```python
from build123d import *

# Parameters (mm, degrees)
SCHIZZO1_R                    = 2
ESTRUSIONE_ESTRUSIONE1_DEPTH  = 3
ESTRUSIONE_ESTRUSIONE2_DEPTH  = 3
SCHIZZO3_W                    = 5
SCHIZZO3_H                    = 5
ESTRUSIONE_ESTRUSIONE3_DEPTH  = 47
SCHIZZO4_R                    = 1.25
TAGLIO_ESTRUSIONE1_DEPTH      = 15
ESTRUSIONE_ESTRUSIONE4_DEPTH  = 5
ESTRUSIONE_ESTRUSIONE5_DEPTH  = 5
SCHIZZO9_W                    = 50
SCHIZZO9_H                    = 46
ESTRUSIONE_ESTRUSIONE8_DEPTH  = 3
SMUSSO1_SIZE                  = 5
SCHIZZO11_W                   = 17
SCHIZZO11_H                   = 46
SCHIZZO11_W_2                 = 64
SCHIZZO11_H_2                 = 58
TAGLIO_ESTRUSIONE3_DEPTH      = 10
SCHIZZO12_W                   = 60
SCHIZZO12_H                   = 20
TAGLIO_ESTRUSIONE4_DEPTH      = 60
SCHIZZO13_W                   = 27
SCHIZZO13_H                   = 46
TAGLIO_ESTRUSIONE5_DEPTH      = 10
RACCORDO1_R                   = 10
SCHIZZO14_W                   = 8
SCHIZZO14_H                   = 14
ESTRUSIONE_ESTRUSIONE9_DEPTH  = 45
SCHIZZO15_R                   = 1.85
TAGLIO_ESTRUSIONE6_DEPTH      = 20
SCHIZZO16_W                   = 8
SCHIZZO16_H                   = 8
ESTRUSIONE_ESTRUSIONE10_DEPTH = 15
SCHIZZO17_R                   = 1.85
TAGLIO_ESTRUSIONE7_DEPTH      = 15
SCHIZZO18_W                   = 8
SCHIZZO18_H                   = 8
ESTRUSIONE_ESTRUSIONE11_DEPTH = 41
SMUSSO3_SIZE                  = 5
SCHIZZO19_W                   = 8
SCHIZZO19_H                   = 58
ESTRUSIONE_ESTRUSIONE12_DEPTH = 3
RACCORDO2_R                   = 10
SCHIZZO20_R                   = 1.85
TAGLIO_ESTRUSIONE8_DEPTH      = 15
SCHIZZO21_W                   = 80
SCHIZZO21_H                   = 6
TAGLIO_ESTRUSIONE9_DEPTH      = 30
SMUSSO4_SIZE                  = 5
ESTRUSIONE_ESTRUSIONE13_DEPTH = 2
SCHIZZO23_W                   = 5
SCHIZZO23_H                   = 2
TAGLIO_ESTRUSIONE10_DEPTH     = 15
SMUSSO5_SIZE                  = 2
ESTRUSIONE_ESTRUSIONE14_DEPTH = 2


with BuildPart() as part:
    # Schizzo1 → Estrusione-Estrusione1 (new body)
    with BuildSketch(Plane.XY):
        with BuildLine():
            Line((4, 70), (4, 27))
            Line((4, 27), (52, 27))
            Line((52, 27), (52, 18))
            Line((52, 18), (4, 18))
            Line((4, 18), (4, -16))
            Line((4, -16), (52, -16))
            Line((52, -16), (52, -24))
            Line((52, -24), (4, -24))
            Line((4, -24), (4, -67))
            ThreePointArc((4, -67), (0, -71), (-4, -67))
            Line((-4, -67), (-4, -24))
            Line((-4, -24), (-52, -24))
            Line((-52, -24), (-52, -16))
            Line((-52, -16), (-4, -16))
            Line((-4, -16), (-4, 18))
            Line((-4, 18), (-52, 18))
            Line((-52, 18), (-52, 27))
            Line((-52, 27), (-4, 27))
            Line((-4, 27), (-4, 70))
            ThreePointArc((-4, 70), (0, 74), (4, 70))
        make_face()
        with Locations((0, 70)):
            Circle(SCHIZZO1_R, mode=Mode.SUBTRACT)
        with Locations((48, 23)):
            Circle(SCHIZZO1_R, mode=Mode.SUBTRACT)
        with Locations((-48, 23)):
            Circle(SCHIZZO1_R, mode=Mode.SUBTRACT)
        with Locations((0, -67)):
            Circle(SCHIZZO1_R, mode=Mode.SUBTRACT)
        with Locations((-48, -20)):
            Circle(SCHIZZO1_R, mode=Mode.SUBTRACT)
        with Locations((48, -20)):
            Circle(SCHIZZO1_R, mode=Mode.SUBTRACT)
    extrude(amount=ESTRUSIONE_ESTRUSIONE1_DEPTH)

    # Schizzo2 → Estrusione-Estrusione2 (add)
    with BuildSketch(Plane.XY):
        Polygon((-42, 57), (-3.921210291, 57), (-3.921210291, 64), (-49, 64), (-49, 26), (-42, 26), align=None)
        Polygon((-49, 4), (-40, 4), (-40, -62), (40, -62), (40, 4), (49, 4), (49, 18), (42, 18), (42, 11), (3.990161704, 11), (3.990161704, 4), (32, 4), (32, -54), (-32, -54), (-32, 4), (-3.921210291, 4), (-3.921210291, 11), (-42, 11), (-42, 18), (-49, 18), align=None)
        Polygon((49, 64), (49, 26), (42, 26), (42, 57), (3.990161704, 57), (3.990161704, 64), align=None)
    extrude(amount=ESTRUSIONE_ESTRUSIONE2_DEPTH)

    # Schizzo3 → Estrusione-Estrusione3 (add)
    with BuildSketch(Plane(origin=(0, 0, 0), x_dir=(-1, 0, 0), z_dir=(0, 0, -1))):
        with Locations((-46.5, 61.5)):
            Rectangle(SCHIZZO3_W, SCHIZZO3_H)
        with Locations((46.5, 61.5)):
            Rectangle(SCHIZZO3_W, SCHIZZO3_H)
        with Locations((46.5, 6.5)):
            Rectangle(SCHIZZO3_W, SCHIZZO3_H)
        with Locations((-46.5, 6.5)):
            Rectangle(SCHIZZO3_W, SCHIZZO3_H)
    extrude(amount=ESTRUSIONE_ESTRUSIONE3_DEPTH)

    # Schizzo4 → Taglio-Estrusione1 (cut)
    with BuildSketch(Plane(origin=(0, 0, -47), x_dir=(-1, 0, 0), z_dir=(0, 0, -1))):
        with Locations((-46.5, 61.5)):
            Circle(SCHIZZO4_R)
        with Locations((46.5, 61.5)):
            Circle(SCHIZZO4_R)
        with Locations((46.5, 6.5)):
            Circle(SCHIZZO4_R)
        with Locations((-46.5, 6.5)):
            Circle(SCHIZZO4_R)
    extrude(amount=-TAGLIO_ESTRUSIONE1_DEPTH, mode=Mode.SUBTRACT)

    # Schizzo5 → Estrusione-Estrusione4 (add)
    with BuildSketch(Plane.XZ.offset(-4)):
        Polygon((-44, 0), (-19, 0), (-44, -29), align=None)
        Polygon((19, 0), (44, 0), (44, -29), align=None)
    extrude(amount=-ESTRUSIONE_ESTRUSIONE4_DEPTH)

    # Schizzo6 → Estrusione-Estrusione5 (add)
    with BuildSketch(Plane(origin=(0, 64, 0), x_dir=(1, 0, 0), z_dir=(0, 1, 0))):
        Polygon((-44, 25), (-19, 0), (-44, 0), align=None)
        Polygon((44, 25), (19, 0), (44, 0), align=None)
    extrude(amount=-ESTRUSIONE_ESTRUSIONE5_DEPTH)

    # Schizzo9 → Estrusione-Estrusione8 (add)
    with BuildSketch(Plane(origin=(0, 0, 0), x_dir=(-1, 0, 0), z_dir=(0, 0, -1))):
        with Locations((0, 34)):
            Rectangle(SCHIZZO9_W, SCHIZZO9_H)
    extrude(amount=-ESTRUSIONE_ESTRUSIONE8_DEPTH)

    # Smusso1
    smusso1_edges = [part.edges().sort_by_distance(p)[0] for p in [
        (4, 64, 1.5),
        (-4, 64, 1.5),
    ]]
    chamfer(smusso1_edges, length=SMUSSO1_SIZE)

    # Schizzo11 → Taglio-Estrusione3 (cut)
    with BuildSketch(Plane(origin=(0, 0, 0), x_dir=(-1, 0, 0), z_dir=(0, 0, -1))):
        with Locations((-33.5, 34)):
            Rectangle(SCHIZZO11_W, SCHIZZO11_H)
        with Locations((33.5, 34)):
            Rectangle(SCHIZZO11_W, SCHIZZO11_H)
        with Locations((0, -25)):
            Rectangle(SCHIZZO11_W_2, SCHIZZO11_H_2)
    extrude(amount=-TAGLIO_ESTRUSIONE3_DEPTH, mode=Mode.SUBTRACT)

    # Schizzo12 → Taglio-Estrusione4 (cut)
    with BuildSketch(Plane.XZ.offset(-4)):
        with Locations((0, -10)):
            Rectangle(SCHIZZO12_W, SCHIZZO12_H)
    extrude(amount=-TAGLIO_ESTRUSIONE4_DEPTH, mode=Mode.SUBTRACT)

    # Schizzo13 → Taglio-Estrusione5 (cut)
    with BuildSketch(Plane(origin=(0, 0, 0), x_dir=(-1, 0, 0), z_dir=(0, 0, -1))):
        with Locations((38.5, 34)):
            Rectangle(SCHIZZO13_W, SCHIZZO13_H)
        with Locations((-38.5, 34)):
            Rectangle(SCHIZZO13_W, SCHIZZO13_H)
    extrude(amount=-TAGLIO_ESTRUSIONE5_DEPTH, mode=Mode.SUBTRACT)

    # Raccordo1
    raccordo1_edges = [part.edges().sort_by_distance(p)[0] for p in [
        (25, 57, 1.5),
        (-25, 11, 1.5),
        (-25, 57, 1.5),
        (25, 11, 1.5),
    ]]
    fillet(raccordo1_edges, radius=RACCORDO1_R)

    # Schizzo14 → Estrusione-Estrusione9 (add)
    with BuildSketch(Plane(origin=(0, 0, 0), x_dir=(-1, 0, 0), z_dir=(0, 0, -1))):
        with Locations((-36, -3)):
            Rectangle(SCHIZZO14_W, SCHIZZO14_H)
        with Locations((36, -3)):
            Rectangle(SCHIZZO14_W, SCHIZZO14_H)
    extrude(amount=ESTRUSIONE_ESTRUSIONE9_DEPTH)

    # Schizzo15 → Taglio-Estrusione6 (cut)
    with BuildSketch(Plane(origin=(0, 0, -45), x_dir=(-1, 0, 0), z_dir=(0, 0, -1))):
        with Locations((36, -6)):
            Circle(SCHIZZO15_R)
        with Locations((-36, -6)):
            Circle(SCHIZZO15_R)
    extrude(amount=-TAGLIO_ESTRUSIONE6_DEPTH, mode=Mode.SUBTRACT)

    # Schizzo16 → Estrusione-Estrusione10 (add)
    with BuildSketch(Plane(origin=(0, 0, 0), x_dir=(-1, 0, 0), z_dir=(0, 0, -1))):
        with Locations((-36, -14)):
            Rectangle(SCHIZZO16_W, SCHIZZO16_H)
        with Locations((36, -14)):
            Rectangle(SCHIZZO16_W, SCHIZZO16_H)
    extrude(amount=ESTRUSIONE_ESTRUSIONE10_DEPTH)

    # Schizzo17 → Taglio-Estrusione7 (cut)
    with BuildSketch(Plane(origin=(0, 0, -15), x_dir=(-1, 0, 0), z_dir=(0, 0, -1))):
        with Locations((-36, -14)):
            Circle(SCHIZZO17_R)
        with Locations((36, -14)):
            Circle(SCHIZZO17_R)
    extrude(amount=-TAGLIO_ESTRUSIONE7_DEPTH, mode=Mode.SUBTRACT)

    # Schizzo18 → Estrusione-Estrusione11 (add)
    with BuildSketch(Plane(origin=(0, 0, 0), x_dir=(-1, 0, 0), z_dir=(0, 0, -1))):
        with Locations((-18, -58)):
            Rectangle(SCHIZZO18_W, SCHIZZO18_H)
        with Locations((18, -58)):
            Rectangle(SCHIZZO18_W, SCHIZZO18_H)
    extrude(amount=ESTRUSIONE_ESTRUSIONE11_DEPTH)

    # Smusso3
    smusso3_edges = [part.edges().sort_by_distance(p)[0] for p in [
        (14, -58, 0),
        (-14, -58, 0),
    ]]
    chamfer(smusso3_edges, length=SMUSSO3_SIZE)

    # Schizzo19 → Estrusione-Estrusione12 (add)
    with BuildSketch(Plane(origin=(0, 0, 0), x_dir=(-1, 0, 0), z_dir=(0, 0, -1))):
        with Locations((0, -25)):
            Rectangle(SCHIZZO19_W, SCHIZZO19_H)
    extrude(amount=-ESTRUSIONE_ESTRUSIONE12_DEPTH)

    # Raccordo2
    raccordo2_edges = [part.edges().sort_by_distance(p)[0] for p in [
        (4, -54, 1.5),
        (-4, -54, 1.5),
        (4, 4, 1.5),
        (-4, 4, 1.5),
    ]]
    fillet(raccordo2_edges, radius=RACCORDO2_R)

    # Schizzo20 → Taglio-Estrusione8 (cut)
    with BuildSketch(Plane(origin=(0, 0, -41), x_dir=(-1, 0, 0), z_dir=(0, 0, -1))):
        with Locations((-18, -58)):
            Circle(SCHIZZO20_R)
        with Locations((18, -58)):
            Circle(SCHIZZO20_R)
    extrude(amount=-TAGLIO_ESTRUSIONE8_DEPTH, mode=Mode.SUBTRACT)

    # Schizzo21 → Taglio-Estrusione9 (cut)
    with BuildSketch(Plane(origin=(0, 0, -45), x_dir=(-1, 0, 0), z_dir=(0, 0, -1))):
        with Locations((0, 1)):
            Rectangle(SCHIZZO21_W, SCHIZZO21_H)
    extrude(amount=-TAGLIO_ESTRUSIONE9_DEPTH, mode=Mode.SUBTRACT)

    # Smusso4
    smusso4_edges = [part.edges().sort_by_distance(p)[0] for p in [
        (-40, 4, -6),
        (40, 4, -6),
    ]]
    chamfer(smusso4_edges, length=SMUSSO4_SIZE)

    # Schizzo22 → Estrusione-Estrusione13 (add)
    with BuildSketch(Plane.XZ.offset(-59)):
        Polygon((49, 0), (30, 0), (30, -11), (44, -25), (44, -47), (49, -47), align=None)
        Polygon((-30, 0), (-49, 0), (-49, -47), (-44, -47), (-44, -25), (-30, -11), align=None)
    extrude(amount=ESTRUSIONE_ESTRUSIONE13_DEPTH)

    # Schizzo23 → Taglio-Estrusione10 (cut)
    with BuildSketch(Plane(origin=(0, 0, -47), x_dir=(-1, 0, 0), z_dir=(0, 0, -1))):
        with Locations((-46.5, 58)):
            Rectangle(SCHIZZO23_W, SCHIZZO23_H)
    extrude(amount=-TAGLIO_ESTRUSIONE10_DEPTH, mode=Mode.SUBTRACT)

    # Smusso5
    smusso5_edges = [part.edges().sort_by_distance(p)[0] for p in [
        (46.5, 59, -32),
    ]]
    chamfer(smusso5_edges, length=SMUSSO5_SIZE - 0.0001)  # a hair under: the kernel refuses the full size

    # Schizzo24 → Estrusione-Estrusione14 (add)
    with BuildSketch(Plane(origin=(0, 9, 0), x_dir=(1, 0, 0), z_dir=(0, 1, 0))):
        Polygon((-49, 0), (-30, 0), (-30, 12.76), (-44, 29), (-44, 47), (-49, 47), align=None)
        Polygon((44, 47), (49, 47), (49, 0), (30, 0), (30, 12.76), (44, 29), align=None)
    extrude(amount=ESTRUSIONE_ESTRUSIONE14_DEPTH)


solid = part.part
```
Check sheet for the modelled part. Datum: model origin and axes. Units: mm. A direction names the side the tool comes from. Round coordinates to 2 decimals unless told otherwise and drop trailing zeros. Write each loop counter-clockwise with the first axis right and the second up, starting at its lowest first coordinate (ties: lowest second). Pieces come first, ordered by that corner, then holes. Notation, with made-up numbers: M 85,63 L 134,63 A24 cw 134,94 Z; hole C 18.25,68.5 d2. An arc over 180 degrees is marked long. Write item = value, one per line. Start each with the question number.
1. Tool access check on faces 1 (the flat face through (-32, -12, -12)), 2 (the flat face through (-36, -10, -30)), 3 (the flat face through (46, -16, 1)). Record the directions out of +Z, -Z, +X, -X, +Y, -Y that give a thin tool (end or side, any length) a straight path to the whole face; none if there is none.
2. Section check C-C, the plane x = 18. Record the cut outline in (y, z), then the cut area to 4 significant figures.
3. Section check B-B, the plane y = -26. Record the cut outline in (x, z).
4. Section check A-A, the plane x = 0. Record the cut outline in (y, z).
5. Scan lines: line 1 (Y direction, x = 48, z = 1); line 2 (Y direction, x = 36, z = -10.25); line 3 (X direction, y = -58, z = -15). Record each from-to range of solid material in increasing order. Write a range as [from, to].
6. Release check for a two-part mould opening along X. For faces 4 (the flat face through (-38, -13, -15)), 5 (the flat face through (37, 61, -18)), 6 (the flat face through (-43, 2, -6)) record: pulls with the +X half, pulls with the -X half, needs draft (parallel to the pull), parting line crosses it, or undercut.
7. Gauge pin test, flat ends, axial feed: pin 1 (5 mm diameter, centred on x = -5, y = 14, fed in from -Z); pin 2 (21 mm diameter, centred on x = 42, z = -7, fed in from -Y); pin 3 (1.5 mm diameter, centred on x = -44.5, z = 1, fed in from +Y). Record the tip position at first contact, or that the pin passes through.
8. Section check D-D, the plane y = 40.5. Record the cut outline in (x, z).
Results found:
q1.face_1 = +Z, -Z
q1.face_2 = -Z, +X, -X, -Y
q1.face_3 = +Z, -Z, +X
q2.outline = M -62,-41 L -59.85,-41 L -59.85,-26 L -56.15,-26 L -56.15,-41 L -54,-41 L -54,3 L -62,3 Z; M 4,0 L 64,0 L 64,3 L 4,3 Z
q2.area = 476.5 mm^2
q3.outline = M -40,0 L -32,0 L -32,3 L -40,3 Z; M -4,0 L 4,0 L 4,3 L -4,3 Z; M 32,0 L 40,0 L 40,3 L 32,3 Z
q4.outline = M -71,0 L -69,0 L -69,3 L -71,3 Z; M -65,0 L 68,0 L 68,3 L -65,3 Z; M 72,0 L 74,0 L 74,3 L 72,3 Z
q5.line_1 = [-24, -22], [-18, -16], [4, 11], [57, 64]
q5.line_2 = [-18, -15.85], [-12.15, 11], [57, 64]
q5.line_3 = [-22, -14], [14, 22]
q6.face_4 = needs draft
q6.face_5 = undercut
q6.face_6 = pulls with the -X half
q7.pin_1 = 0
q7.pin_2 = -62
q7.pin_3 = 64
q8.outline = M -25,0 L 25,0 L 25,3 L -25,3 Z
